Verification items for the finished model (mm, model axes). A direction names the side the tool comes from. Round coordinates to 2 decimals unless told otherwise and drop trailing zeros. Order: outer loops, then holes, each group sorted by start corner. A loop starts at its lowest first (then second) coordinate and runs counter-clockwise, first axis right, second up.
```python
from build123d import *

# Parameters (mm, degrees)
SKETCH1_W                        = 6.35
SKETCH1_H                        = 6.35
BOSS_EXTRUDE1_DEPTH              = 6.35
F_1_8_0_125_DIAMETER_HOLE1_D     = 3.175
F_1_8_0_125_DIAMETER_HOLE1_DEPTH = 70.104
F_1_8_0_125_DIAMETER_HOLE1_TIP   = 0.953866233
SKETCH4_W                        = 5.334
SKETCH4_H                        = 5.842
CUT_EXTRUDE1_DEPTH               = 11.998522628
F_1_8_0_125_DIAMETER_HOLE2_D     = 3.175
F_1_8_0_125_DIAMETER_HOLE2_DEPTH = 70.104
F_1_8_0_125_DIAMETER_HOLE2_TIP   = 0.953866233


with BuildPart() as part:
    # Sketch1 → Boss-Extrude1 (new body)
    with BuildSketch(Plane(origin=(0, 0, 0), x_dir=(0, 0, -1), z_dir=(1, 0, 0))):
        with Locations((3.175, 3.175)):
            Rectangle(SKETCH1_W, SKETCH1_H)
    extrude(amount=BOSS_EXTRUDE1_DEPTH)

    # 1/8 (0.125) Diameter Hole1
    with Locations(Plane(origin=(6.35, 0, 0), x_dir=(0, 0, -1), z_dir=(1, 0, 0))):
        with Locations((3.175, 3.175)):
            Hole(F_1_8_0_125_DIAMETER_HOLE1_D / 2, depth=F_1_8_0_125_DIAMETER_HOLE1_DEPTH)
            with Locations((0, 0, -(F_1_8_0_125_DIAMETER_HOLE1_DEPTH + F_1_8_0_125_DIAMETER_HOLE1_TIP / 2))):  # 118° drill point
                Cone(0, F_1_8_0_125_DIAMETER_HOLE1_D / 2, F_1_8_0_125_DIAMETER_HOLE1_TIP, mode=Mode.SUBTRACT)

    # Sketch4 → Cut-Extrude1 (cut, through all)
    with BuildSketch(Plane(origin=(0, 0, -6.35), x_dir=(-1, 0, 0), z_dir=(0, 0, -1))):
        with Locations((-3.175, 3.429)):
            Rectangle(SKETCH4_W, SKETCH4_H)
    extrude(amount=-CUT_EXTRUDE1_DEPTH, mode=Mode.SUBTRACT)

    # 1/8 (0.125) Diameter Hole2
    with Locations(Plane(origin=(0, 0, 0), x_dir=(-1, 0, 0), z_dir=(0, -1, 0))):
        with Locations((-3.175, 3.175)):
            Hole(F_1_8_0_125_DIAMETER_HOLE2_D / 2, depth=F_1_8_0_125_DIAMETER_HOLE2_DEPTH)
            with Locations((0, 0, -(F_1_8_0_125_DIAMETER_HOLE2_DEPTH + F_1_8_0_125_DIAMETER_HOLE2_TIP / 2))):  # 118° drill point
                Cone(0, F_1_8_0_125_DIAMETER_HOLE2_D / 2, F_1_8_0_125_DIAMETER_HOLE2_TIP, mode=Mode.SUBTRACT)


solid = part.part
```
1) Scan lines: probe 1 along X at (y, z) = (5.5, -3.75); probe 2 along Y at (x, z) = (1.5, -5.5); probe 3 along Z at (x, y) = (6, 2.5). Record each from-to range of solid material in increasing order.
2) Draft check along Z on faces 3 (the flat face through (3.4, 0.3, 0)), 4 (the flat face through (6.35, 5, -2)), 5 (the flat face through (3.4, 0.3, -6.35)), 6 (the cylindrical face through (0.3, 4.5, -2.3)). Enter one of: released by +Z, released by -Z, zero draft, split by the parting line, or undercut.
3) Tool access check on faces 1 (the flat face through (5.842, 5, -3)), 2 (the flat face through (1.7, 0, -1.7)). Record the directions out of +Z, -Z, +X, -X, +Y, -Y that give a thin tool (end or side, any length) a straight path to the whole face; none if there is none.
4) Sectioned sample at C-C on x = 4. Record the cut outline in (y, z), then the cut area to 3 significant figures.
5) Sectioned sample at D-D on y = 4.25. Record the cut outline in (x, z).
6) Go/stop test with a flat-tipped pin: pin 1 Ø3 at (y, z) = (4.5, -3) entering from +X. Record where the tip stops, or that it passes through.
7) Sectioned sample at B-B on z = -3. Record the cut outline in (x, y), then the cut area to 3 significant figures.
8) Sectioned sample at A-A on y = 5.5. Record the cut outline in (x, z), then the cut area to 3 significant figures.
Returned:
1. probe 1: x = 0 to 0.51, 5.84 to 6.35
1. probe 2: y = 0 to 0.51
1. probe 3: z = -6.35 to -4.61, -1.74 to 0
2. face 3: released by +Z
2. face 4: zero draft
2. face 5: released by -Z
2. face 6: undercut
3. face 1: +Z, -Z, +Y
3. face 2: +Z, -Z, +X, -X, -Y
4. outline: (0, -6.35) - (0.51, -6.35) - (0.51, -4.53) - (0, -4.53) - close; (0, -1.82) - (0.51, -1.82) - (0.51, 0) - (0, 0) - close
4. area: 1.85 mm2
5. outline: (0, -6.35) - (0.51, -6.35) - (0.51, -4.34) - (0, -4.34) - close; (0, -2.01) - (0.51, -2.01) - (0.51, 0) - (0, 0) - close; (5.84, -6.35) - (6.35, -6.35) - (6.35, -4.34) - (5.84, -4.34) - close; (5.84, -2.01) - (6.35, -2.01) - (6.35, 0) - (5.84, 0) - close
6. pin 1: stops at x = 6.35
7. outline: (0, 0) - (1.6, 0) - (1.6, 0.51) - (0.51, 0.51) - (0.51, 1.6) - (0, 1.6) - close; (0, 4.75) - (0.51, 4.75) - (0.51, 6.35) - (0, 6.35) - close; (4.75, 0) - (6.35, 0) - (6.35, 1.6) - (5.84, 1.6) - (5.84, 0.51) - (4.75, 0.51) - close; (5.84, 4.75) - (6.35, 4.75) - (6.35, 6.35) - (5.84, 6.35) - close
7. area: 4.35 mm2
8. outline: (0, -6.35) - (0.51, -6.35) - (0.51, 0) - (0, 0) - close; (5.84, -6.35) - (6.35, -6.35) - (6.35, 0) - (5.84, 0) - close
8. area: 6.45 mm2
